from build123d import *

# Parameters (mm, degrees)
SKETCH1_W           = 42.3
SKETCH1_H           = 15.6
BOSS_EXTRUDE1_DEPTH = 3
SKETCH2_R           = 1
CUT_EXTRUDE1_DEPTH  = 4
SKETCH3_R           = 3.5
CUT_EXTRUDE2_DEPTH  = 4
CUT_EXTRUDE3_DEPTH  = 4


with BuildPart() as part:
    # Sketch1 → Boss-Extrude1 (new body)
    with BuildSketch(Plane.XY):
        with Locations((21.15, 7.8)):
            Rectangle(SKETCH1_W, SKETCH1_H)
    extrude(amount=BOSS_EXTRUDE1_DEPTH)

    # Sketch2 → Cut-Extrude1 (cut, through all)
    with BuildSketch(Plane.XY.offset(3)):
        with Locations((2, 13.6)):
            Circle(SKETCH2_R)
        with Locations((40.3, 13.6)):
            Circle(SKETCH2_R)
        with Locations((40.3, 2)):
            Circle(SKETCH2_R)
        with Locations((2, 2)):
            Circle(SKETCH2_R)
    extrude(amount=-CUT_EXTRUDE1_DEPTH, mode=Mode.SUBTRACT)

    # Sketch3 → Cut-Extrude2 (cut, through all)
    with BuildSketch(Plane.XY.offset(3)):
        with Locations((16, 9.55)):
            Circle(SKETCH3_R)
    extrude(amount=-CUT_EXTRUDE2_DEPTH, mode=Mode.SUBTRACT)

    # Sketch4 → Cut-Extrude3 (cut, through all)
    with BuildSketch(Plane.XY.offset(3)):
        with BuildLine():
            Line((12, 0), (20, 0))
            ThreePointArc((20, 0), (16, 2.438447187), (12, 0))
        make_face()
    extrude(amount=-CUT_EXTRUDE3_DEPTH, mode=Mode.SUBTRACT)


solid = part.part
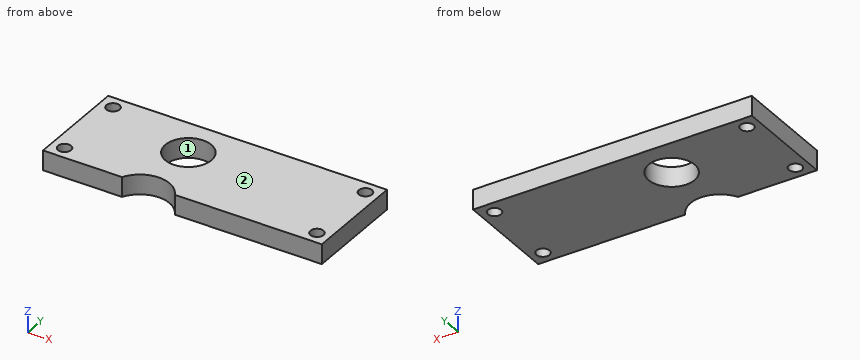
The listing builds one solid part. Answer for the finished solid, in the listing's coordinates (mm). Face numbers are marked on the shaded views. Give positions to 0.01 mm unless a question says otherwise; leave off trailing zeros. Write each loop counter-clockwise with the first axis right and the second up, starting at its lowest first coordinate (ties: lowest second). Pieces come first, ordered by that corner, then holes.
Item 1: Section C-C, the plane z = 2.5 is taken. Write down the section's boundary in (x, y).
Item 2: Find the intervals of material crossed by line 1 along Y through (x, z) = (2, 1); line 2 along Y through (x, z) = (16, 0.85); line 3 along Y through (x, z) = (14, 1.2), in increasing order.
Item 3: Flat-ended cylindrical pins translate along their axes: P1, Ø1.2, axis at x = 2, y = 2, coming from the -Z side; P2, Ø8, axis at x = 19.5, y = 4.5, coming from the -Z side. Find the tip coordinate at first contact, or state that the pin passes through.
Item 4: Section A-A, the plane y = 13.6 is taken. Write down the section's boundary in (x, z).
Item 5: Determine the mould class of the marked faces 1 and 2 for opening direction X: released by +X, released by -X, zero draft, split by the parting line, or undercut.
Item 6: Section B-B, the plane x = 16 is taken. Write down the section's boundary in (y, z), plus the area to 3 significant figures.
Item 7: Section D-D, the plane x = 40.3 is taken. Write down the section's boundary in (y, z), plus the area to 3 significant figures.
Completed:
1. outline: (0, 0) - (12, 0) arc R4.5 cw to (20, 0) - (42.3, 0) - (42.3, 15.6) - (0, 15.6) - close; hole circle Ø2 at (2, 2); hole circle Ø2 at (2, 13.6); hole circle Ø7 at (16, 9.55); hole circle Ø2 at (40.3, 2); hole circle Ø2 at (40.3, 13.6)
2. line 1: y = 0 to 1, 3 to 12.6, 14.6 to 15.6
2. line 2: y = 2.44 to 6.05, 13.05 to 15.6
2. line 3: y = 1.97 to 6.68, 12.42 to 15.6
3. P1: passes through
3. P2: stops at z = 0
4. outline: (0, 0) - (1, 0) - (1, 3) - (0, 3) - close; (3, 0) - (39.3, 0) - (39.3, 3) - (3, 3) - close; (41.3, 0) - (42.3, 0) - (42.3, 3) - (41.3, 3) - close
5. face 1: undercut
5. face 2: zero draft
6. outline: (2.44, 0) - (6.05, 0) - (6.05, 3) - (2.44, 3) - close; (13.05, 0) - (15.6, 0) - (15.6, 3) - (13.05, 3) - close
6. area: 18.5 mm2
7. outline: (0, 0) - (1, 0) - (1, 3) - (0, 3) - close; (3, 0) - (12.6, 0) - (12.6, 3) - (3, 3) - close; (14.6, 0) - (15.6, 0) - (15.6, 3) - (14.6, 3) - close
7. area: 34.8 mm2
